```python
from build123d import *

# Parameters (mm, degrees)
F0_W     = 44.45
F0_H     = 101.6
F1_DEPTH = 44.45
F2_R     = 6.35
F3_DEPTH = 59.69
F4_R     = 5.08
F5_R     = 5.08


with BuildPart() as f1:
    # F0 (on Top) → F1 (new body)
    with BuildSketch(Plane.XY):
        with Locations((22.225, -50.8)):
            Rectangle(F0_W, F0_H)
    extrude(amount=F1_DEPTH)

    # F2 (on face) → F3 (cut)
    with BuildSketch(Plane.XY.offset(44.45)):
        with Locations((22.225, -12.7)):
            Circle(F2_R)
        with Locations((22.225, -88.9)):
            Circle(F2_R)
    extrude(amount=-F3_DEPTH, mode=Mode.SUBTRACT)

    # F4
    f4_edges = [f1.edges().sort_by_distance(p)[0] for p in [
        (44.45, -50.8, 44.45),
        (44.45, -50.8, 0),
        (0, -50.8, 0),
        (0, -50.8, 44.45),
    ]]
    fillet(f4_edges, radius=F4_R)

    # F5
    f5_edges = [f1.edges().sort_by_distance(p)[0] for p in [
        (44.45, 0, 22.225),
        (42.962102, 0, 1.487898),
        (42.962102, 0, 42.962102),
        (22.225, 0, 0),
        (22.225, 0, 44.45),
        (1.487898, 0, 1.487898),
        (1.487898, 0, 42.962102),
        (0, 0, 22.225),
        (0, -101.6, 22.225),
        (1.487898, -101.6, 1.487898),
        (1.487898, -101.6, 42.962102),
        (22.225, -101.6, 0),
        (22.225, -101.6, 44.45),
        (42.962102, -101.6, 1.487898),
        (42.962102, -101.6, 42.962102),
        (44.45, -101.6, 22.225),
    ]]
    fillet(f5_edges, radius=F5_R)


solid = f1.part
```
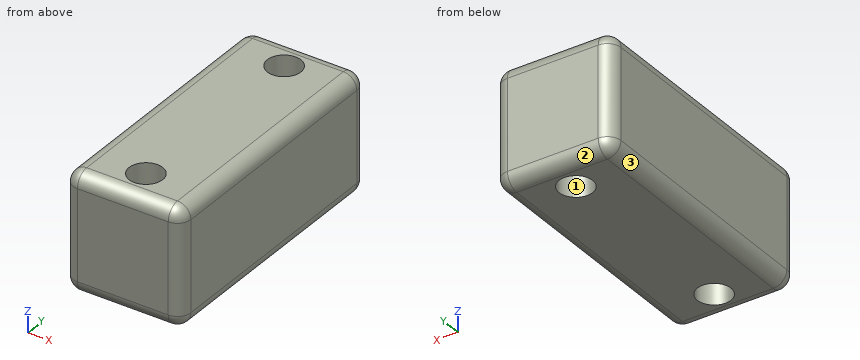
Verification items for the finished model (mm, model axes). Face numbers are marked on the shaded views. Round coordinates to 2 decimals unless told otherwise and drop trailing zeros. Write each loop counter-clockwise with the first axis right and the second up, starting at its lowest first coordinate (ties: lowest second). Pieces come first, ordered by that corner, then holes. Notation, with made-up numbers: (53, 10.25) - (88, 10.25) arc R20 cw to (88, 46.25) - close; hole circle Ø5 at (8.25, 4). An arc over 180 degrees is marked (long way). Answer as a JSON object with one key per item and string values. Group by question number.
Q1. Section check A-A, the plane y = -12.7. Enter the section's corners in (x, z) (3 decimals).
Q2. Go/stop test with a flat-tipped pin: pin 1 Ø11.5 at (x, y) = (22.225, -88.9) entering from +Z. Record where the tip stops, or that it passes through.
Q3. Section check B-B, the plane x = 23. Enter the section's corners in (y, z).
Q4. Mould release check, pull along X, two halves, no side actions. Record for the marked faces 1, 2 and 3: released by +X, released by -X, zero draft, split by the parting line, or undercut.
Q5. Thickness scan on line 1 (Y direction, x = 23, z = 11); line 2 (Y direction, x = 23.5, z = 35); line 3 (X direction, y = -88, z = 3.5). Record the ranges inside material, lowest first.
Q6. Section check C-C, the plane z = 10. Enter the section's corners in (x, y) (3 decimals).
Q7. Section check D-D, the plane y = -92.5. Enter the section's corners in (x, z), plus the area to 3 significant figures.
Found:
{
 "1": {"outline": "(0, 5.08) arc R5.08 ccw to (5.08, 0) - (15.875, 0) - (15.875, 44.45) - (5.08, 44.45) arc R5.08 ccw to (0, 39.37) - close; (28.575, 0) - (39.37, 0) arc R5.08 ccw to (44.45, 5.08) - (44.45, 39.37) arc R5.08 ccw to (39.37, 44.45) - (28.575, 44.45) - close"},
 "2": {"pin 1": "passes through"},
 "3": {"outline": "(-101.6, 5.08) arc R5.08 ccw to (-96.52, 0) - (-95.2, 0) - (-95.2, 44.45) - (-96.52, 44.45) arc R5.08 ccw to (-101.6, 39.37) - close; (-82.6, 0) - (-19, 0) - (-19, 44.45) - (-82.6, 44.45) - close; (-6.4, 0) - (-5.08, 0) arc R5.08 ccw to (0, 5.08) - (0, 39.37) arc R5.08 ccw to (-5.08, 44.45) - (-6.4, 44.45) - close"},
 "4": {"face 1": "undercut", "face 2": "zero draft", "face 3": "released by -X"},
 "5": {"line 1": "y = -101.6 to -95.2, -82.6 to -19, -6.4 to 0", "line 2": "y = -101.6 to -95.12, -82.68 to -18.92, -6.48 to 0", "line 3": "x = 0.25 to 15.94, 28.51 to 44.2"},
 "6": {"outline": "(0, -96.52) arc R5.08 ccw to (5.08, -101.6) - (39.37, -101.6) arc R5.08 ccw to (44.45, -96.52) - (44.45, -5.08) arc R5.08 ccw to (39.37, 0) - (5.08, 0) arc R5.08 ccw to (0, -5.08) - close; hole circle Ø12.7 at (22.225, -88.9); hole circle Ø12.7 at (22.225, -12.7)"},
 "7": {"outline": "(0, 5.08) arc R5.08 ccw to (5.08, 0) - (16.99, 0) - (16.99, 44.45) - (5.08, 44.45) arc R5.08 ccw to (0, 39.37) - close; (27.46, 0) - (39.37, 0) arc R5.08 ccw to (44.45, 5.08) - (44.45, 39.37) arc R5.08 ccw to (39.37, 44.45) - (27.46, 44.45) - close", "area": "1,490 mm^2"}
}
